Here's the drawing with two shaded views (mm, measured from the low corner). I have some questions. Give positions to 0.01 mm unless a question says otherwise; leave off trailing zeros. Order: outer loops, then holes, each group sorted by start corner. A loop starts at its lowest first (then second) coordinate and runs counter-clockwise, first axis right, second up. Notation, with made-up numbers: M 10,11 L 16,11 A19 ccw 16,43 Z; hole C -26.5,78 d11. An arc over 180 degrees is marked long. Use a Markdown table: item, result. Add a question column.
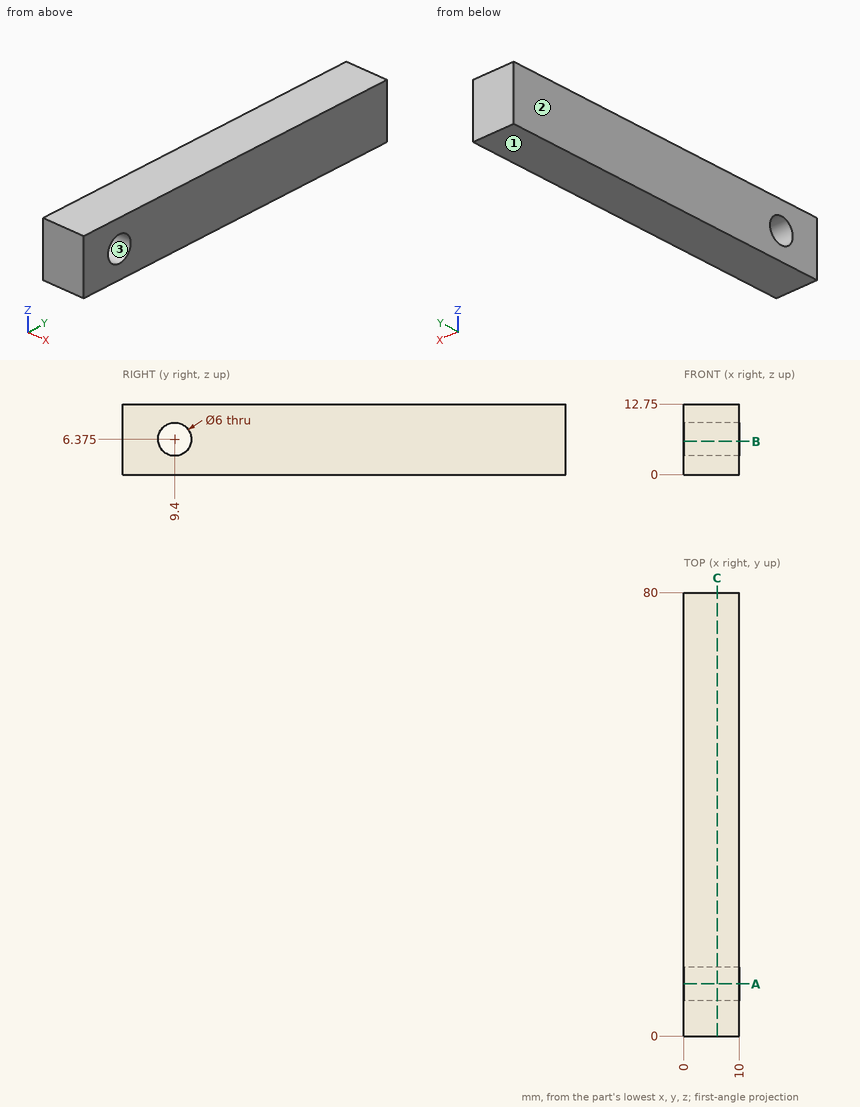
1. If we section it at C-C, the plane x = 6: List the corners of the cut face in (y, z) for me (3 decimals).
2. We'd pull the mould along Z, two halves only. Please class the marked faces 1, 2 and 3: +Z half, -Z half, draft (parallel to the pull), parting line (faces both ways), or undercut.
3. I need wall thicknesses on L1, parallel to Z at x = 1, y = 9.5; L2, parallel to Y at x = 9, z = 4.5; L3, parallel to Y at x = 2.75, z = 5.5. Which ranges of each line are inside material? Lowest first, please. Write a range as [from, to].
4. If we section it at B-B, the plane z = 6: List the corners of the cut face in (x, y) for me, then the cut area to 3 significant figures.
5. If we section it at A-A, the plane y = 9.4: List the corners of the cut face in (x, z) for me (3 decimals).
Geometry results:
| question | item | result |
|---|---|---|
| 1 | outline | M 0,0 L 80,0 L 80,12.75 L 0,12.75 Z; hole C 9.4,6.375 d6 |
| 2 | face 1 | -Z half |
| 2 | face 2 | draft |
| 2 | face 3 | undercut |
| 3 | L1 | z = [0, 3.38], [9.37, 12.75] |
| 3 | L2 | y = [0, 7.06], [11.74, 80] |
| 3 | L3 | y = [0, 6.53], [12.27, 80] |
| 4 | outline | M 0,0 L 10,0 L 10,6.42 L 0,6.42 Z; M 0,12.38 L 10,12.38 L 10,80 L 0,80 Z |
| 4 | area | 740 mm^2 |
| 5 | outline | M 0,0 L 10,0 L 10,3.375 L 0,3.375 Z; M 0,9.375 L 10,9.375 L 10,12.75 L 0,12.75 Z |
